Build history of the part. All positions in model axes, mm. Face numbers are marked on the shaded views. A direction names the side the tool comes from. Round coordinates to 2 decimals unless told otherwise and drop trailing zeros. Loops run counter-clockwise (first coordinate to the right, second up) from the corner with the lowest first, then second, coordinate; pieces in that order, holes last. Notation, with made-up numbers: M 21,2.25 L 56,2.25 A23 ccw 56,38.25 Z; hole C 16.25,-23 d9. An arc over 180 degrees is marked long. One line per item, written item: value.
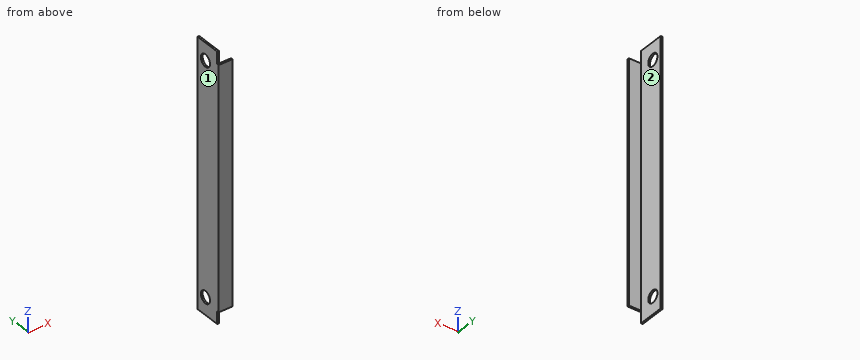
Autodesk Inventor part; units mm, degrees
ref_plane "YZ Plane" through (0, 0, 0) normal (1, 0, 0) x (0, 1, 0)
ref_plane "XZ Plane" through (0, 0, 0) normal (0, 1, 0) x (-1, 0, 0)
ref_plane "XY Plane" through (0, 0, 0) normal (0, 0, 1) x (1, 0, 0)
sketch "Sketch1" plane through (0, 0, 0) normal (0, 0, 1) x (1, 0, 0)
  line L0 (0, 0) -> (25.4, 0)
  line L1 (25.4, 0) -> (25.4, 3.175)
  line L2 (3.175, 50.8) -> (0, 50.8)
  line L3 (0, 50.8) -> (0, 0)
  line L4 (3.175, 50.8) -> (3.175, 3.175)
  line L5 (3.175, 3.175) -> (25.4, 3.175)
  dimension "d0" = 50.8
  dimension "d1" = 25.4
  dimension "d2" = 3.175
  dimension "d3" = 3.175
extrude "Extrusion1" add sketch "Sketch1" along normal blind 482.6
sketch "Sketch2" plane through (0, 0, 0) normal (-1, 0, 0) x (0, 0, 1)
  line L0 (482.6, 0) -> (482.6, 50.8)
  line L1 (0, 0) -> (482.6, 0)
  circle A0 centre (450.85, 31.75) radius 11.1125
  line L2 (0, 50.8) -> (0, 0)
  circle A1 centre (31.75, 31.75) radius 11.1125
  dimension "d6" = 22.225
  dimension "d7" = 31.75
  dimension "d8" = 31.75
  dimension "d17" = 31.75
  dimension "d18" = 31.75
extrude "Extrusion2" cut sketch "Sketch2" against normal blind 508
sketch "Sketch3" plane through (0, 0, 0) normal (0, -1, 0) x (1, 0, 0)
  line L0 (0, 0) -> (0, 482.6)
  line L1 (0, 0) -> (25.4, 0)
  line L2 (25.4, 0) -> (25.4, 482.6)
  line L3 (0, 22.225) -> (25.4, 22.225)
  line L4 (25.4, 482.6) -> (0, 482.6)
  line L5 (0, 460.375) -> (25.4, 460.375)
  dimension "d13" = 22.225
  dimension "d16" = 22.225
extrude "Extrusion3" cut sketch "Sketch3" against normal blind 3.175 contours L0 L3 L2 L1 | L0 L4 L2 L5
equation "\"d3\" = d2"
equation "\"d17\" = d8"
equation "\"d18\" = d7"
equation "\"d16\" = d13"
properties part number "manipulator L frame middle"
Item 1: Which spindle directions (+Z, -Z, +X, -X, +Y, -Y) get a long thin tool onto all of the face, cutting with end or side? Do the marked faces 1 and 2. Say none if no direction does.
Check values:
face 1: +Z, -Z, -X, +Y, -Y
face 2: +Z, -Z, +X, +Y
Item 2: Slice it at D-D, the plane x = 7. Give the cut face in (y, z) (3 decimals).
Check values:
outline: M 0,22.225 L 3.175,22.225 L 3.175,460.375 L 0,460.375 Z
Item 3: Slice it at A-A, the plane z = 31.75. Give the cut face in (x, y) (1 decimal).
Check values:
outline: M 0,0 L 25.4,0 L 25.4,3.2 L 3.2,3.2 L 3.2,20.6 L 0,20.6 Z; M 0,42.9 L 3.2,42.9 L 3.2,50.8 L 0,50.8 Z
Item 4: Drop flat-ended pins along their axis: P1, Ø3.5, axis at x = 13.5, y = 2, coming from the +Z side (3 decimals); P2, Ø24, axis at y = 29.5, z = 129, coming from the +X side (3 decimals); P3, Ø2, axis at x = 14.5, z = 245, coming from the +Y side (3 decimals). Give the stop position or say it passes through.
Check values:
P1: stops at z = 460.375
P2: stops at x = 3.175
P3: stops at y = 3.175
Item 5: Slice it at B-B, the plane y = 31.75. Give the cut face in (x, z) (1 decimal).
Check values:
outline: M 0,0 L 3.2,0 L 3.2,20.6 L 0,20.6 Z; M 0,42.9 L 3.2,42.9 L 3.2,439.7 L 0,439.7 Z; M 0,462 L 3.2,462 L 3.2,482.6 L 0,482.6 Z
Item 6: Slice it at C-C, the plane z = 376.5. Give the cut face in (x, y) (3 decimals).
Check values:
outline: M 0,0 L 25.4,0 L 25.4,3.175 L 3.175,3.175 L 3.175,50.8 L 0,50.8 Z
Item 7: Wall check: line 1 along Y through (x, z) = (0.9, 450.85); line 2 along Y through (x, z) = (14.75, 319.5) (3 decimals). Give the ranges that are in metal, low to high.
Check values:
line 1: y = 0 to 20.64, 42.86 to 50.8
line 2: y = 0 to 3.175
